```python
from build123d import *

# Parameters (mm, degrees)
SKETCH2_W                   = 38.1
SKETCH2_H                   = 38.1
BOSS_EXTRUDE1_DEPTH         = 170.686028715
SKETCH3_W                   = 157.986028715
SKETCH3_H                   = 31.75
CUT_EXTRUDE1_DEPTH          = 17.4625
FILLET1_R                   = 3.175
FILLET1_OF_MIRROR1_R        = 3.175
F_1_4_0_25_DIAMETER_HOLE1_D = 6.35
CUT_EXTRUDE2_REACH          = 178.1
FILLET3_R                   = 3.175


with BuildPart() as part:
    # Sketch2 → Boss-Extrude1 (new body)
    with BuildSketch(Plane.XY):
        with Locations((19.05, 19.05)):
            Rectangle(SKETCH2_W, SKETCH2_H)
    extrude(amount=BOSS_EXTRUDE1_DEPTH)

    # Sketch3 → Cut-Extrude1 (cut)
    with BuildSketch(Plane(origin=(38.1, 0, 0), x_dir=(0, 0, -1), z_dir=(1, 0, 0))):
        with Locations((-85.343014357, 19.05)):
            Rectangle(SKETCH3_W, SKETCH3_H)
    cut_extrude1 = extrude(amount=-CUT_EXTRUDE1_DEPTH, mode=Mode.SUBTRACT)

    # Fillet1
    fillet1_edges = [part.edges().sort_by_distance(p)[0] for p in [
        (29.36875, 3.175, 164.336028715),
        (29.36875, 34.925, 164.336028715),
        (29.36875, 34.925, 6.35),
        (29.36875, 3.175, 6.35),
    ]]
    fillet(fillet1_edges, radius=FILLET1_R)

    # Mirror1: Cut-Extrude1 across plane
    add(cut_extrude1.mirror(Plane(origin=(19.05, 0, 0), x_dir=(0, 0, 1), z_dir=(1, 0, 0))), mode=Mode.SUBTRACT)

    # Fillet1 of Mirror1
    fillet1_of_mirror1_edges = [part.edges().sort_by_distance(p)[0] for p in [
        (8.73125, 3.175, 164.336028715),
        (8.73125, 34.925, 164.336028715),
        (8.73125, 34.925, 6.35),
        (8.73125, 3.175, 6.35),
    ]]
    fillet(fillet1_of_mirror1_edges, radius=FILLET1_OF_MIRROR1_R)

    # 1/4 (0.25) Diameter Hole1 (through all)
    with Locations(Plane(origin=(0, 0, 0), x_dir=(-1, 0, 0), z_dir=(0, 0, -1))):
        with Locations((-9.525, 25.4), (-9.525, 12.7), (-28.575, 12.7), (-28.575, 25.4)):
            Hole(F_1_4_0_25_DIAMETER_HOLE1_D / 2)

    # Sketch7 → Cut-Extrude2 (cut, up to next)
    with BuildSketch(Plane.ZY.offset(-17.4625), mode=Mode.PRIVATE) as cut_extrude2_sk1:
        Polygon((12.7, 31.75), (12.7, 6.35), (46.354412352, 6.35), align=None)
    cut_extrude2_tool1 = extrude(cut_extrude2_sk1.sketch, amount=-CUT_EXTRUDE2_REACH, mode=Mode.PRIVATE) & part.part
    # Sketch7 → Cut-Extrude2 (cut, up to next)
    with BuildSketch(Plane.ZY.offset(-17.4625), mode=Mode.PRIVATE) as cut_extrude2_sk2:
        Polygon((23.240930553, 31.75), (56.895342905, 6.35), (56.895342905, 31.75), align=None)
    cut_extrude2_tool2 = extrude(cut_extrude2_sk2.sketch, amount=-CUT_EXTRUDE2_REACH, mode=Mode.PRIVATE) & part.part
    # Sketch7 → Cut-Extrude2 (cut, up to next)
    with BuildSketch(Plane.ZY.offset(-17.4625), mode=Mode.PRIVATE) as cut_extrude2_sk3:
        Polygon((63.245342905, 31.75), (63.245342905, 6.35), (96.899755257, 6.35), align=None)
    cut_extrude2_tool3 = extrude(cut_extrude2_sk3.sketch, amount=-CUT_EXTRUDE2_REACH, mode=Mode.PRIVATE) & part.part
    # Sketch7 → Cut-Extrude2 (cut, up to next)
    with BuildSketch(Plane.ZY.offset(-17.4625), mode=Mode.PRIVATE) as cut_extrude2_sk4:
        Polygon((73.786273458, 31.75), (107.44068581, 6.35), (107.44068581, 31.75), align=None)
    cut_extrude2_tool4 = extrude(cut_extrude2_sk4.sketch, amount=-CUT_EXTRUDE2_REACH, mode=Mode.PRIVATE) & part.part
    # Sketch7 → Cut-Extrude2 (cut, up to next)
    with BuildSketch(Plane.ZY.offset(-17.4625), mode=Mode.PRIVATE) as cut_extrude2_sk5:
        Polygon((113.79068581, 31.75), (113.79068581, 6.35), (147.445098162, 6.35), align=None)
    cut_extrude2_tool5 = extrude(cut_extrude2_sk5.sketch, amount=-CUT_EXTRUDE2_REACH, mode=Mode.PRIVATE) & part.part
    # Sketch7 → Cut-Extrude2 (cut, up to next)
    with BuildSketch(Plane.ZY.offset(-17.4625), mode=Mode.PRIVATE) as cut_extrude2_sk6:
        Polygon((124.331616363, 31.75), (157.986028715, 6.35), (157.986028715, 31.75), align=None)
    cut_extrude2_tool6 = extrude(cut_extrude2_sk6.sketch, amount=-CUT_EXTRUDE2_REACH, mode=Mode.PRIVATE) & part.part
    add(cut_extrude2_tool1.solids().sort_by_distance((17.4625, 14.816667, 23.918137))[0], mode=Mode.SUBTRACT)
    add(cut_extrude2_tool2.solids().sort_by_distance((17.4625, 23.283333, 45.677205))[0], mode=Mode.SUBTRACT)
    add(cut_extrude2_tool3.solids().sort_by_distance((17.4625, 14.816667, 74.46348))[0], mode=Mode.SUBTRACT)
    add(cut_extrude2_tool4.solids().sort_by_distance((17.4625, 23.283333, 96.222548))[0], mode=Mode.SUBTRACT)
    add(cut_extrude2_tool5.solids().sort_by_distance((17.4625, 14.816667, 125.008823))[0], mode=Mode.SUBTRACT)
    add(cut_extrude2_tool6.solids().sort_by_distance((17.4625, 23.283333, 146.767891))[0], mode=Mode.SUBTRACT)

    # Fillet3
    fillet3_edges = [part.edges().sort_by_distance(p)[0] for p in [
        (19.05, 31.75, 12.7),
        (19.05, 6.35, 46.354412352),
        (19.05, 6.35, 12.7),
        (19.05, 31.75, 23.240930553),
        (19.05, 31.75, 56.895342905),
        (19.05, 6.35, 56.895342905),
        (19.05, 31.75, 63.245342905),
        (19.05, 6.35, 96.899755257),
        (19.05, 6.35, 63.245342905),
        (19.05, 31.75, 113.79068581),
        (19.05, 6.35, 147.445098162),
        (19.05, 6.35, 113.79068581),
        (19.05, 31.75, 73.786273458),
        (19.05, 31.75, 107.44068581),
        (19.05, 6.35, 107.44068581),
        (19.05, 31.75, 124.331616363),
        (19.05, 31.75, 157.986028715),
        (19.05, 6.35, 157.986028715),
    ]]
    fillet(fillet3_edges, radius=FILLET3_R)


solid = part.part
```
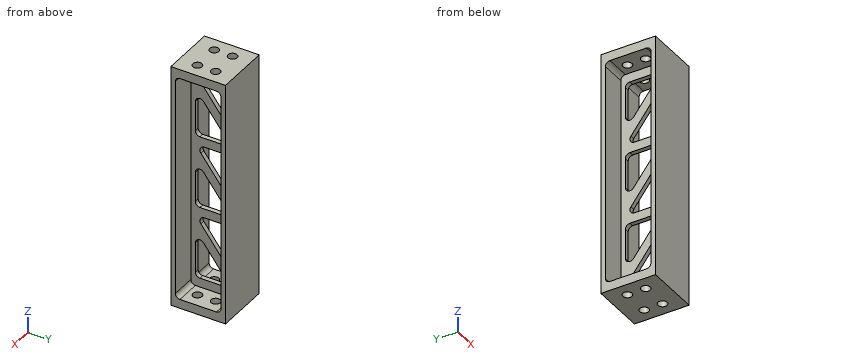
For this review, take the finished solid that the model builds, in its own axes (mm). Coordinates: 2 decimals unless noted, no trailing zeros. Order: outer loops, then holes, each group sorted by start corner. A loop starts at its lowest first (then second) coordinate and runs counter-clockwise, first axis right, second up. Notation, with made-up numbers: (19.25, 55.25) -> (26.25, 55.25) arc R7 cw to (26.25, 68.25) -> close; hole circle Ø4 at (36, -8). An arc over 180 degrees is marked (long way). Use CSV: the item, a comma, the result in double quotes. Start each with the question number.
Item 1: Wall thickness on probe 1 along X at (y, z) = (25, 2); probe 2 along Y at (x, z) = (26, 92) (3 decimals); probe 3 along Z at (x, y) = (22, 21): over which ranges is each line inside the solid? List them lowest first.
Item 2: Insertion check: pin 1 (12 mm diameter, centred on y = 19, z = 72, fed in from +X). The pin has a flat end and moves straight along its axis. Give the tip position at first contact, or say it passes through.
Item 3: We need section A-A, the plane x = 34. Give the boundary of the cut face in (y, z) (3 decimals), then the cut area to 3 significant figures.
Derived:
1,probe 1,"x = 0 to 6.38, 12.67 to 25.43, 31.72 to 38.1"
1,probe 2,"y = 0 to 3.175, 34.925 to 38.1"
1,probe 3,"z = 0 to 6.35, 164.34 to 170.69"
2,pin 1,"stops at x = 20.64"
3,outline,"(0, 0) -> (38.1, 0) -> (38.1, 170.686) -> (0, 170.686) -> close; hole (3.175, 9.525) arc R3.175 ccw to (6.35, 6.35) -> (31.75, 6.35) arc R3.175 ccw to (34.925, 9.525) -> (34.925, 161.161) arc R3.175 ccw to (31.75, 164.336) -> (6.35, 164.336) arc R3.175 ccw to (3.175, 161.161) -> close"
3,area,"1,500 mm^2"
